Model file for the job. Use its own axes, mm. Face numbers are marked on the shaded views. A direction names the side the tool comes from. Give positions to 0.01 mm unless a question says otherwise; leave off trailing zeros. Order: outer loops, then holes, each group sorted by start corner. A loop starts at its lowest first (then second) coordinate and runs counter-clockwise, first axis right, second up. Notation, with made-up numbers: (-29.75, 59.25) - (0.25, 59.25) arc R32 cw to (0.25, 90.25) - close; hole circle Ø6 at (63, -2.5). An arc over 180 degrees is marked (long way). Return JSON: item names as keys, results as strings. Group by question number.
from build123d import *

# Parameters (mm, degrees)
SALIENTE_EXTRUIR1_DEPTH = 2
CORTAR_EXTRUIR1_REACH   = 13.628
CORTAR_EXTRUIR2_REACH   = 13.628
SALIENTE_EXTRUIR3_DEPTH = 3
REDONDEO3_R             = 0.5
REDONDEO4_R             = 1


with BuildPart() as part:
    # Croquis1 → Saliente-Extruir1 (new body)
    with BuildSketch(Plane.XY):
        with BuildLine():
            Line((8.1, 0), (8.1, -5))
            Line((8.1, -5), (-8.1, -5))
            Line((-8.1, -5), (-8.1, 0))
            ThreePointArc((-8.1, 0), (0, 8.1), (8.1, 0))
        make_face()
    extrude(amount=SALIENTE_EXTRUIR1_DEPTH)

    # Croquis4 → Cortar-Extruir1 (cut, up to next)
    with BuildSketch(Plane.XY.offset(2), mode=Mode.PRIVATE) as cortar_extruir1_sk1:
        with BuildLine():
            Line((-1.532970972, 2.1), (1.532970972, 2.1))
            ThreePointArc((1.532970972, 2.1), (0, -2.6), (-1.532970972, 2.1))
        make_face()
    cortar_extruir1_tool1 = extrude(cortar_extruir1_sk1.sketch, amount=-CORTAR_EXTRUIR1_REACH, mode=Mode.PRIVATE) & part.part
    add(cortar_extruir1_tool1.solids().sort_by_distance((0, -0.118931, 2))[0], mode=Mode.SUBTRACT)

    # Croquis5 → Cortar-Extruir2 (cut, up to next)
    with BuildSketch(Plane.XY.offset(2), mode=Mode.PRIVATE) as cortar_extruir2_sk1:
        with BuildLine():
            Line((-4.1, -5), (-4.1, 6.985699679))
            ThreePointArc((-4.1, 6.985699679), (-7.029224708, 4.024922359), (-8.1, 0))
            Line((-8.1, 0), (-8.1, -5))
            Line((-8.1, -5), (-4.1, -5))
        make_face()
    cortar_extruir2_tool1 = extrude(cortar_extruir2_sk1.sketch, amount=-CORTAR_EXTRUIR2_REACH, mode=Mode.PRIVATE) & part.part
    add(cortar_extruir2_tool1.solids().sort_by_distance((-5.920703, 0.103857, 2))[0], mode=Mode.SUBTRACT)

    # Croquis7 → Saliente-Extruir3 (add)
    with BuildSketch(Plane.XY.offset(2)):
        with BuildLine():
            Line((8.1, 0), (8.1, -5))
            Line((8.1, -5), (7.1, -5))
            Line((7.1, -5), (7.1, 0))
            ThreePointArc((7.1, 0), (5.020457997, 5.020458296), (-4.23e-07, 7.1))
            Line((-4.23e-07, 7.1), (-4.23e-07, 8.1))
            ThreePointArc((-4.23e-07, 8.1), (5.727564778, 5.727565077), (8.1, 0))
        make_face()
    extrude(amount=SALIENTE_EXTRUIR3_DEPTH)

    # Redondeo3
    redondeo3_edges = [part.edges().sort_by_distance(p)[0] for p in [
        (5.727564778, 5.727565077, 5),
        (5.020457997, 5.020458296, 5),
        (7.1, -2.5, 5),
        (8.1, -2.5, 5),
    ]]
    fillet(redondeo3_edges, radius=REDONDEO3_R - 0.0001)  # a hair under: the kernel refuses the full size

    # Redondeo4
    redondeo4_edges = [part.edges().sort_by_distance(p)[0] for p in [
        (-4.1, -5, 1),
        (-4.1, 6.985699679, 1),
        (-4.23e-07, 7.6, 2),
    ]]
    fillet(redondeo4_edges, radius=REDONDEO4_R)


solid = part.part
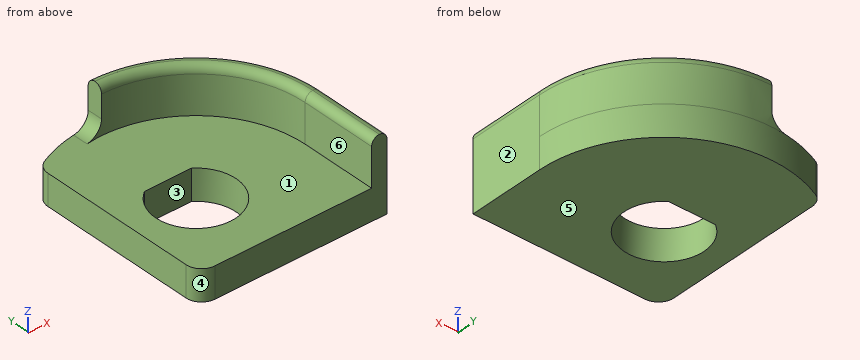
(1) Pull direction X, two halves, no side cores. Call the marked faces 1, 2, 3 and 4: released by +X, released by -X, zero draft, split by the parting line, or undercut.
(2) Drill centre lines: L1, parallel to Y at x = 0, z = 1.2; L2, parallel to Z at x = 4.75, y = -2.25; L3, parallel to X at y = -2, z = 0.9. Where is each one in solid material? Low to high.
(3) 3-axis set-ups, long thin cutter, end or side, ignore diameter. For the marked faces 5 and 6: which of +Z, -Z, +X, -X, +Y, -Y reach the whole face in a straight line?
(4) Drop flat-ended pins along their axis: pin 1 Ø1.3 at (y, z) = (-1.5, 4) entering from -X; pin 2 Ø3 at (y, z) = (3.5, 4.5) entering from -X; pin 3 Ø2 at (x, z) = (2.5, 1) entering from +Y. Give the stop position or say it passes through.
(5) Slice it at C-C (z = 3.9). Give the cut face in (x, y).
(6) Slice it at D-D (z = 2.65). Give the cut face in (x, y).
Result set:
{
 "1": {"face 1": "zero draft", "face 2": "released by +X", "face 3": "undercut", "face 4": "released by -X"},
 "2": {"L1": "y = -5 to -2.6, 2.1 to 8.1", "L2": "z = 0 to 2", "L3": "x = -4.1 to -1.66, 1.66 to 8.1"},
 "3": {"face 5": "-Z, +X, -X, +Y, -Y", "face 6": "+Z, -X, -Y"},
 "4": {"pin 1": "stops at x = 7.1", "pin 2": "stops at x = 5.04", "pin 3": "stops at y = 7.96"},
 "5": {"outline": "(0, 7.1) arc R7.1 cw to (7.1, 0) - (7.1, -5) - (8.1, -5) - (8.1, 0) arc R8.1 ccw to (0, 8.1) - close"},
 "6": {"outline": "(-0.06, 7.1) arc R7.1 cw to (7.1, 0) - (7.1, -5) - (8.1, -5) - (8.1, 0) arc R8.1 ccw to (-0.06, 8.1) - close"}
}
